Can you work these out from the model? Positions are in its coordinate system, mm. Face numbers are marked on the shaded views. A direction names the side the tool comes from. Coordinates: 2 decimals unless noted, no trailing zeros. Order: outer loops, then holes, each group sorted by start corner. A loop starts at its lowest first (then second) coordinate and runs counter-clockwise, first axis right, second up. Notation, with made-up numbers: (11.5, 0) -> (18.5, 0) arc R14 ccw to (18.5, 16) -> close; hole circle Ø3 at (-13, 76.5). An arc over 180 degrees is marked (long way). Return JSON: item names as keys, results as strings. Group by question number.
1) For pin 1 (4 mm diameter, centred on x = 40, y = 15, fed in from -Z); pin 2 (1.5 mm diameter, centred on x = 36.5, z = 1.5, fed in from -Y), each with a flat end and sliding along its axis, tell me the tip position at first contact or that it passes through.
2) If we section it at C-C, the plane z = 2.4: Please give me the cut outline in (x, y), then the cut area to 3 significant figures.
3) If I drill on probe 1 along X at (y, z) = (10.5, 0.95); probe 2 along X at (y, z) = (22.25, 1.25); probe 3 along Y at (x, z) = (36, 1.3), over which ranges is the centre line in solid material (lowest first)? Write a range as from..to.
4) Thinking about a two-plate mould opening in Y: for the marked faces 1, 2, 3 and 4, which applies, +Y half, -Y half, draft (parallel to the pull), parting line (faces both ways), or undercut?
5) If we section it at B-B, the plane y = 17.5: Please give me the cut outline in (x, z).
6) For the marked faces 5, 6, 7 and 8, which set-ups out of +Z, -Z, +X, -X, +Y, -Y let a thin tool reach every point of the face, with its end or its side?
7) If we section it at A-A, the plane x = 37.5: Please give me the cut outline in (y, z), then the cut area to 3 significant figures.
8) If we section it at D-D, the plane x = 29: Please give me the cut outline in (y, z).
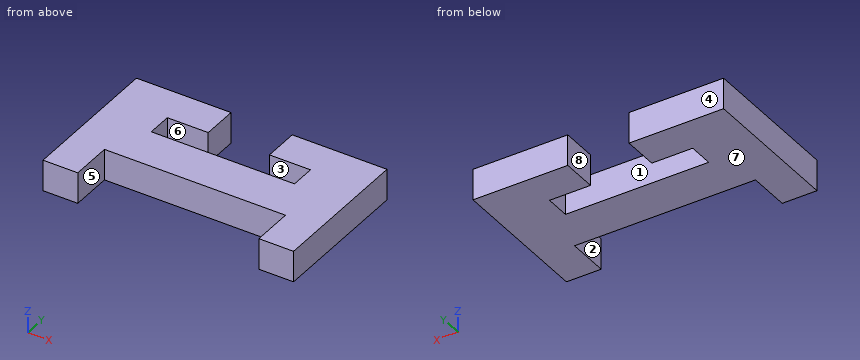
from build123d import *

# Parameters (mm, degrees)
SALIENTE_EXTRUIR1_DEPTH = 3


with BuildPart() as part:
    # Model → Saliente-Extruir1 (new body)
    with BuildSketch(Plane.XY):
        Polygon((31.7, 16.782683294), (24.293333333, 16.782683294), (24.293333333, 19.182683294), (28.24, 19.182683294), (28.24, 22.6), (19.113333333, 22.6), (19.113333333, 8.6), (22.468, 8.6), (22.468, 12.6), (39.932, 12.6), (39.932, 8.6), (43.286666667, 8.6), (43.286666667, 22.6), (34.14656693, 22.6), (34.14656693, 19.182683294), (38.106666667, 19.182683294), (38.106666667, 16.782683294), align=None)
    extrude(amount=SALIENTE_EXTRUIR1_DEPTH)


solid = part.part
Result sheet:
{
 "1": {"pin 1": "stops at z = 0", "pin 2": "stops at y = 12.6"},
 "2": {"outline": "(19.11, 8.6) -> (22.47, 8.6) -> (22.47, 12.6) -> (39.93, 12.6) -> (39.93, 8.6) -> (43.29, 8.6) -> (43.29, 22.6) -> (34.15, 22.6) -> (34.15, 19.18) -> (38.11, 19.18) -> (38.11, 16.78) -> (24.29, 16.78) -> (24.29, 19.18) -> (28.24, 19.18) -> (28.24, 22.6) -> (19.11, 22.6) -> close", "area": "215 mm2"},
 "3": {"probe 1": "x = 19.11..22.47, 39.93..43.29", "probe 2": "x = 19.11..28.24, 34.15..43.29", "probe 3": "y = 12.6..16.78, 19.18..22.6"},
 "4": {"face 1": "undercut", "face 2": "draft", "face 3": "undercut", "face 4": "+Y half"},
 "5": {"outline": "(19.11, 0) -> (24.29, 0) -> (24.29, 3) -> (19.11, 3) -> close; (38.11, 0) -> (43.29, 0) -> (43.29, 3) -> (38.11, 3) -> close"},
 "6": {"face 5": "+Z, -Z, -Y", "face 6": "+Z, -Z", "face 7": "-Z, +X, -X, +Y, -Y", "face 8": "+Z, -Z, +Y"},
 "7": {"outline": "(12.6, 0) -> (16.78, 0) -> (16.78, 3) -> (12.6, 3) -> close; (19.18, 0) -> (22.6, 0) -> (22.6, 3) -> (19.18, 3) -> close", "area": "22.8 mm2"},
 "8": {"outline": "(12.6, 0) -> (16.78, 0) -> (16.78, 3) -> (12.6, 3) -> close"}
}
